from build123d import *

# Parameters (mm, degrees)
F0_W     = 0.0285906434
F0_H     = 5
F0_W_2   = 28.72
F0_R     = 1.8
F0_W_3   = 57.44
F1_DEPTH = 3
F2_R     = 2.5
F3_SIZE  = 0.75


# Not quite as in the source:
# - a feature names something its author has since deleted; it is built from what else it names


with BuildPart() as f1:
    # F0 (on Front) → F1 (new body)
    with BuildSketch(Plane.XZ):
        with Locations((-28.7342953217, 18.525)):
            Rectangle(F0_W, F0_H)
        with Locations((28.7342953217, 18.525)):
            Rectangle(F0_W, F0_H)
        with Locations((-14.36, 18.525)):
            Rectangle(F0_W_2, F0_H)
        with Locations((14.36, 18.525)):
            Rectangle(F0_W_2, F0_H)
        with Locations((14.36, 42.9671912789)):
            Rectangle(F0_W_2, F0_H)
        Polygon((28.72, 94.9421003461), (28.72, 74.9421003461), (28.72, 69.9421003461), (28.72, 45.4671912789), (28.72, 40.4671912789), (28.72, 21.025), (28.7485906434, 21.025), (28.7485906434, 16.025), (28.72, 16.025), (28.72, -3.975), (37.32, -3.975), (37.32, 94.9421003461), align=None)
        with Locations((33.02, 0.325)):
            Circle(F0_R, mode=Mode.SUBTRACT)
        with Locations((33.02, 46.1421912789)):
            Circle(F0_R, mode=Mode.SUBTRACT)
        with Locations((33.02, 60.325)):
            Circle(F0_R, mode=Mode.SUBTRACT)
        with Locations((33.02, 88.0521912789)):
            Circle(F0_R, mode=Mode.SUBTRACT)
        with Locations((-14.36, 42.9671912789)):
            Rectangle(F0_W_2, F0_H)
        Polygon((-28.72, 94.9421003461), (-37.32, 94.9421003461), (-37.32, -3.975), (-28.72, -3.975), (-28.72, 16.025), (-28.7485906434, 16.025), (-28.7485906434, 21.025), (-28.72, 21.025), (-28.72, 40.4671912789), (-28.72, 45.4671912789), (-28.72, 69.9421003461), (-28.72, 74.9421003461), align=None)
        with Locations((-33.02, 0.325)):
            Circle(F0_R, mode=Mode.SUBTRACT)
        with Locations((-33.02, 42.3821003461)):
            Circle(F0_R, mode=Mode.SUBTRACT)
        with Locations((-33.02, 60.325)):
            Circle(F0_R, mode=Mode.SUBTRACT)
        with Locations((-33.02, 90.6421003461)):
            Circle(F0_R, mode=Mode.SUBTRACT)
        with Locations((0, 72.4421003461)):
            Rectangle(F0_W_3, F0_H)
    extrude(amount=F1_DEPTH)

    # F2
    f2_edges = [f1.edges().sort_by_distance(p)[0] for p in [
        (-28.72, -1.5, 45.467191),
        (28.72, -1.5, 45.467191),
        (-28.72, -1.5, 40.467191),
        (28.72, -1.5, 40.467191),
        (-28.72, -1.5, 21.025),
        (28.72, -1.5, 21.025),
        (-28.72, -1.5, 16.025),
        (28.72, -1.5, 16.025),
        (28.72, -1.5, -3.975),
        (37.32, -1.5, -3.975),
        (-37.32, -1.5, -3.975),
        (-28.72, -1.5, -3.975),
        (37.32, -1.5, 94.9421),
        (28.72, -1.5, 94.9421),
        (-37.32, -1.5, 94.9421),
        (-28.72, -1.5, 94.9421),
        (-28.72, -1.5, 69.9421),
        (28.72, -1.5, 69.9421),
        (-28.72, -1.5, 74.9421),
        (28.72, -1.5, 74.9421),
    ]]
    fillet(f2_edges, radius=F2_R)

    # F3
    f3_edges = [f1.edges().sort_by_distance(p)[0] for p in [
        (0, 0, 16.025),
        (0, 0, 40.467191),
        (-33.02, -3, 94.9421),
        (0, -3, 40.467191),
        (0, -3, 69.9421),
        (0, 0, 69.9421),
    ]]
    chamfer(f3_edges, length=F3_SIZE)


solid = f1.part
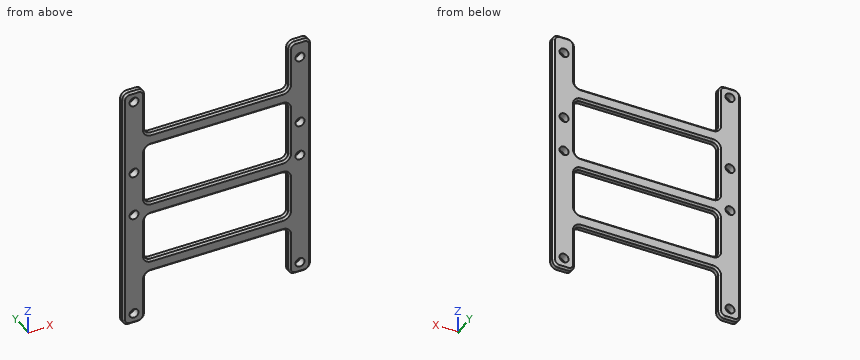
Part model, mm, in its own coordinate system. Round coordinates to 2 decimals unless told otherwise and drop trailing zeros. Order: outer loops, then holes, each group sorted by start corner. A loop starts at its lowest first (then second) coordinate and runs counter-clockwise, first axis right, second up. Notation, with made-up numbers: (59, 84) -> (80, 84) arc R20 cw to (80, 106) -> close; hole circle Ø2 at (-19.75, 87). An arc over 180 degrees is marked (long way). Put each result on its own line as item: value.
Q1. Pin check, flat tips, straight feed: pin 1 Ø2 at (x, z) = (33.02, 60.325) entering from +Y (1 decimal); pin 2 Ø1.2 at (x, y) = (-7.5, -2) entering from +Z; pin 3 Ø0.8 at (x, y) = (-9.5, -1.5) entering from -Z (3 decimals). Stop position of each tip, or through.
From the geometry:
pin 1: passes through
pin 2: stops at z = 74.94
pin 3: stops at z = 16.025
Q2. Band-saw the part on B-B (x = -8.5). Give the cut face in (y, z) (3 decimals).
From the geometry:
outline: (-3, 16.775) -> (-2.25, 16.025) -> (-0.75, 16.025) -> (0, 16.775) -> (0, 20.275) -> (-0.75, 21.025) -> (-2.25, 21.025) -> (-3, 20.275) -> close; (-3, 41.217) -> (-2.25, 40.467) -> (-0.75, 40.467) -> (0, 41.217) -> (0, 44.717) -> (-0.75, 45.467) -> (-2.25, 45.467) -> (-3, 44.717) -> close; (-3, 70.692) -> (-2.25, 69.942) -> (-0.75, 69.942) -> (0, 70.692) -> (0, 74.192) -> (-0.75, 74.942) -> (-2.25, 74.942) -> (-3, 74.192) -> close
Q3. Wall check: line 1 (Z direction, x = 33.02, y = -0.9) (3 decimals); line 2 (Z direction, x = -7, y = -1.85) (3 decimals); line 3 (Z direction, x = -33.02, y = -0.9) (3 decimals). Give the ranges that are in metal, low to high. Write a range as [from, to].
From the geometry:
line 1: z = [-3.975, -1.475], [2.125, 44.342], [47.942, 58.525], [62.125, 86.252], [89.852, 94.942]
line 2: z = [16.025, 21.025], [40.467, 45.467], [69.942, 74.942]
line 3: z = [-3.975, -1.475], [2.125, 40.582], [44.182, 58.525], [62.125, 88.842], [92.442, 94.942]
Q4. Band-saw the part on C-C (y = -1.75). State how many separate pieces and enclosed holes the cut face has, and give its area (3 significant figures).
From the geometry:
separate pieces: 1
enclosed holes: 10
area: 2,490 mm2
Q5. Band-saw the part on A-A (x = -33.02). Give the cut face in (y, z) (3 decimals), and give its area (3 significant figures).
From the geometry:
outline: (-3, -3.225) -> (-2.25, -3.975) -> (-0.75, -3.975) -> (0, -3.225) -> (0, -1.475) -> (-3, -1.475) -> close; (-3, 2.125) -> (0, 2.125) -> (0, 40.582) -> (-3, 40.582) -> close; (-3, 44.182) -> (0, 44.182) -> (0, 58.525) -> (-3, 58.525) -> close; (-3, 62.125) -> (0, 62.125) -> (0, 88.842) -> (-3, 88.842) -> close; (-3, 92.442) -> (0, 92.442) -> (0, 94.192) -> (-0.75, 94.942) -> (-2.25, 94.942) -> (-3, 94.192) -> close
area: 252 mm2
